```python
from build123d import *

# Parameters (mm, degrees)
SKETCH1_W           = 240
SKETCH1_H           = 130
SKETCH1_W_2         = 3.175
SKETCH1_H_2         = 4
SKETCH1_W_3         = 20
SKETCH1_H_3         = 3.175
SKETCH1_W_4         = 4
BOSS_EXTRUDE1_DEPTH = 3.175
SKETCH2_W           = 240.08128
SKETCH2_H           = 130.08128
SKETCH2_W_2         = 3.91872
SKETCH2_H_2         = 3.09372
SKETCH2_W_3         = 3.09372
SKETCH2_H_3         = 3.91872
SKETCH2_W_4         = 19.91872
BOSS_EXTRUDE2_DEPTH = 3.175


with BuildPart() as part:
    # Sketch1 → Boss-Extrude1 (new body)
    with BuildSketch(Plane(origin=(0, 0, 0), x_dir=(1, 0, 0), z_dir=(0, 1, 0))):
        Rectangle(SKETCH1_W, SKETCH1_H)
        with Locations((-111.5875, -50)):
            Rectangle(SKETCH1_W_2, SKETCH1_H_2, mode=Mode.SUBTRACT)
        with Locations((-100, -56.5875)):
            Rectangle(SKETCH1_W_3, SKETCH1_H_3, mode=Mode.SUBTRACT)
        with Locations((-60, -56.5875)):
            Rectangle(SKETCH1_W_3, SKETCH1_H_3, mode=Mode.SUBTRACT)
        with Locations((-20, -56.5875)):
            Rectangle(SKETCH1_W_3, SKETCH1_H_3, mode=Mode.SUBTRACT)
        with Locations((-11.5, -23.4125)):
            Rectangle(SKETCH1_W_4, SKETCH1_H_3, mode=Mode.SUBTRACT)
        with Locations((-66.5, -23.4125)):
            Rectangle(SKETCH1_W_4, SKETCH1_H_3, mode=Mode.SUBTRACT)
        with Locations((-55, -23.4125)):
            Rectangle(SKETCH1_W_4, SKETCH1_H_3, mode=Mode.SUBTRACT)
        with Locations((-43.5, -23.4125)):
            Rectangle(SKETCH1_W_4, SKETCH1_H_3, mode=Mode.SUBTRACT)
        with Locations((-35.4375, -15.35)):
            Rectangle(SKETCH1_W_2, SKETCH1_H_2, mode=Mode.SUBTRACT)
        with Locations((-35.4375, -3.85)):
            Rectangle(SKETCH1_W_2, SKETCH1_H_2, mode=Mode.SUBTRACT)
        with Locations((-35.4375, 7.65)):
            Rectangle(SKETCH1_W_2, SKETCH1_H_2, mode=Mode.SUBTRACT)
        with Locations((-43.5, 15.7125)):
            Rectangle(SKETCH1_W_4, SKETCH1_H_3, mode=Mode.SUBTRACT)
        with Locations((-55, 15.7125)):
            Rectangle(SKETCH1_W_4, SKETCH1_H_3, mode=Mode.SUBTRACT)
        with Locations((-66.5, 15.7125)):
            Rectangle(SKETCH1_W_4, SKETCH1_H_3, mode=Mode.SUBTRACT)
        with Locations((-74.5625, 7.65)):
            Rectangle(SKETCH1_W_2, SKETCH1_H_2, mode=Mode.SUBTRACT)
        with Locations((-74.5625, -3.85)):
            Rectangle(SKETCH1_W_2, SKETCH1_H_2, mode=Mode.SUBTRACT)
        with Locations((-74.5625, -15.35)):
            Rectangle(SKETCH1_W_2, SKETCH1_H_2, mode=Mode.SUBTRACT)
        with Locations((20, -56.5875)):
            Rectangle(SKETCH1_W_3, SKETCH1_H_3, mode=Mode.SUBTRACT)
        with Locations((60, -56.5875)):
            Rectangle(SKETCH1_W_3, SKETCH1_H_3, mode=Mode.SUBTRACT)
        with Locations((100, -56.5875)):
            Rectangle(SKETCH1_W_3, SKETCH1_H_3, mode=Mode.SUBTRACT)
        with Locations((111.5875, -50)):
            Rectangle(SKETCH1_W_2, SKETCH1_H_2, mode=Mode.SUBTRACT)
        with Locations((0, -23.4125)):
            Rectangle(SKETCH1_W_4, SKETCH1_H_3, mode=Mode.SUBTRACT)
        with Locations((11.5, -23.4125)):
            Rectangle(SKETCH1_W_4, SKETCH1_H_3, mode=Mode.SUBTRACT)
        with Locations((43.5, -23.4125)):
            Rectangle(SKETCH1_W_4, SKETCH1_H_3, mode=Mode.SUBTRACT)
        with Locations((55, -23.4125)):
            Rectangle(SKETCH1_W_4, SKETCH1_H_3, mode=Mode.SUBTRACT)
        with Locations((66.5, -23.4125)):
            Rectangle(SKETCH1_W_4, SKETCH1_H_3, mode=Mode.SUBTRACT)
        with Locations((-111.5875, 50)):
            Rectangle(SKETCH1_W_2, SKETCH1_H_2, mode=Mode.SUBTRACT)
        with Locations((-105, 56.5875)):
            Rectangle(SKETCH1_W_4, SKETCH1_H_3, mode=Mode.SUBTRACT)
        with Locations((105, 56.5875)):
            Rectangle(SKETCH1_W_4, SKETCH1_H_3, mode=Mode.SUBTRACT)
        with Locations((111.5875, 50)):
            Rectangle(SKETCH1_W_2, SKETCH1_H_2, mode=Mode.SUBTRACT)
    extrude(amount=BOSS_EXTRUDE1_DEPTH)

    # Sketch2 → Boss-Extrude2 (add)
    with BuildSketch(Plane(origin=(0, 3.175, 0), x_dir=(1, 0, 0), z_dir=(0, 1, 0))):
        Rectangle(SKETCH2_W, SKETCH2_H)
        with Locations((-105, 56.5875)):
            Rectangle(SKETCH2_W_2, SKETCH2_H_2, mode=Mode.SUBTRACT)
        with Locations((-74.5625, -3.85)):
            Rectangle(SKETCH2_W_3, SKETCH2_H_3, mode=Mode.SUBTRACT)
        with Locations((-35.4375, 7.65)):
            Rectangle(SKETCH2_W_3, SKETCH2_H_3, mode=Mode.SUBTRACT)
        with Locations((-111.5875, 50)):
            Rectangle(SKETCH2_W_3, SKETCH2_H_3, mode=Mode.SUBTRACT)
        with Locations((-74.5625, -15.35)):
            Rectangle(SKETCH2_W_3, SKETCH2_H_3, mode=Mode.SUBTRACT)
        with Locations((105, 56.5875)):
            Rectangle(SKETCH2_W_2, SKETCH2_H_2, mode=Mode.SUBTRACT)
        with Locations((-11.5, -23.4125)):
            Rectangle(SKETCH2_W_2, SKETCH2_H_2, mode=Mode.SUBTRACT)
        with Locations((111.5875, 50)):
            Rectangle(SKETCH2_W_3, SKETCH2_H_3, mode=Mode.SUBTRACT)
        with Locations((-66.5, 15.7125)):
            Rectangle(SKETCH2_W_2, SKETCH2_H_2, mode=Mode.SUBTRACT)
        with Locations((-35.4375, -3.85)):
            Rectangle(SKETCH2_W_3, SKETCH2_H_3, mode=Mode.SUBTRACT)
        with Locations((-111.5875, -50)):
            Rectangle(SKETCH2_W_3, SKETCH2_H_3, mode=Mode.SUBTRACT)
        with Locations((-55, 15.7125)):
            Rectangle(SKETCH2_W_2, SKETCH2_H_2, mode=Mode.SUBTRACT)
        with Locations((-100, -56.5875)):
            Rectangle(SKETCH2_W_4, SKETCH2_H_2, mode=Mode.SUBTRACT)
        with Locations((-35.4375, -15.35)):
            Rectangle(SKETCH2_W_3, SKETCH2_H_3, mode=Mode.SUBTRACT)
        with Locations((-60, -56.5875)):
            Rectangle(SKETCH2_W_4, SKETCH2_H_2, mode=Mode.SUBTRACT)
        with Locations((-43.5, 15.7125)):
            Rectangle(SKETCH2_W_2, SKETCH2_H_2, mode=Mode.SUBTRACT)
        with Locations((-20, -56.5875)):
            Rectangle(SKETCH2_W_4, SKETCH2_H_2, mode=Mode.SUBTRACT)
        with Locations((0, -23.4125)):
            Rectangle(SKETCH2_W_2, SKETCH2_H_2, mode=Mode.SUBTRACT)
        with Locations((20, -56.5875)):
            Rectangle(SKETCH2_W_4, SKETCH2_H_2, mode=Mode.SUBTRACT)
        with Locations((-66.5, -23.4125)):
            Rectangle(SKETCH2_W_2, SKETCH2_H_2, mode=Mode.SUBTRACT)
        with Locations((60, -56.5875)):
            Rectangle(SKETCH2_W_4, SKETCH2_H_2, mode=Mode.SUBTRACT)
        with Locations((-55, -23.4125)):
            Rectangle(SKETCH2_W_2, SKETCH2_H_2, mode=Mode.SUBTRACT)
        with Locations((100, -56.5875)):
            Rectangle(SKETCH2_W_4, SKETCH2_H_2, mode=Mode.SUBTRACT)
        with Locations((11.5, -23.4125)):
            Rectangle(SKETCH2_W_2, SKETCH2_H_2, mode=Mode.SUBTRACT)
        with Locations((-43.5, -23.4125)):
            Rectangle(SKETCH2_W_2, SKETCH2_H_2, mode=Mode.SUBTRACT)
        with Locations((111.5875, -50)):
            Rectangle(SKETCH2_W_3, SKETCH2_H_3, mode=Mode.SUBTRACT)
        with Locations((-74.5625, 7.65)):
            Rectangle(SKETCH2_W_3, SKETCH2_H_3, mode=Mode.SUBTRACT)
        with Locations((43.5, -23.4125)):
            Rectangle(SKETCH2_W_2, SKETCH2_H_2, mode=Mode.SUBTRACT)
        with Locations((55, -23.4125)):
            Rectangle(SKETCH2_W_2, SKETCH2_H_2, mode=Mode.SUBTRACT)
        with Locations((66.5, -23.4125)):
            Rectangle(SKETCH2_W_2, SKETCH2_H_2, mode=Mode.SUBTRACT)
    extrude(amount=-BOSS_EXTRUDE2_DEPTH)


solid = part.part
```
The listing builds one solid part. Answer for the finished solid, in the listing's coordinates (mm). Coordinates: 2 decimals unless noted, no trailing zeros. Loops run counter-clockwise (first coordinate to the right, second up) from the corner with the lowest first, then second, coordinate; pieces in that order, holes last. Notation, with made-up numbers: (18.25, 32) - (51.25, 32) arc R21 cw to (51.25, 43) - close; hole circle Ø9 at (-22, 62). An arc over 180 degrees is marked (long way). Write item = value, one per line.
1) Find the intervals of material crossed by line 1 along Z through (x, y) = (10.5, 1.85); line 2 along Z through (x, y) = (-42, 1.9); line 3 along X through (y, z) = (2.3, 2), in increasing order.
Responses:
line_1 = -65.04 to 21.87, 24.96 to 55.04, 58.13 to 65.04
line_2 = -65.04 to -17.26, -14.17 to 21.87, 24.96 to 65.04
line_3 = -120.04 to -76.11, -73.02 to -36.98, -33.89 to 120.04
2) Section B-B (y = 1.2) is taken. Count the separate pieces of the cut face and the enclosed holes in it, plus the area to 3 significant figures.
Responses:
separate_pieces = 1
enclosed_holes = 30
area = 30,600 mm^2
3) This flat-tipped pin is pushed along its axis until it touches: P1, Ø8, axis at x = 71, z = 34.5, coming from the -Y side. Where does it stop, or does it pass through?
Responses:
P1 = 0
4) Section A-A (x = -95.5) is taken. Determine the outline of the cut face in (y, z) (3 decimals), plus the area to 3 significant figures.
Responses:
outline = (0, -65.041) - (3.175, -65.041) - (3.175, 55.041) - (0, 55.041) - close; (0, 58.134) - (3.175, 58.134) - (3.175, 65.041) - (0, 65.041) - close
area = 403 mm^2
